Design review of the part shown in the three views and the two pictorial views. Dimensions are in mm from the part's minimum x, y and z. A direction names the side the tool comes from. Coordinates: 2 decimals unless noted, no trailing zeros. Loops run counter-clockwise (first coordinate to the right, second up) from the corner with the lowest first, then second, coordinate; pieces in that order, holes last. Notation, with made-up numbers: M 14.5,-31.75 L 56.5,-31.75 A19 ccw 56.5,-11.75 Z; hole C 17.5,41 d9. An arc over 180 degrees is marked long. Answer as a JSON object with one key per item and string values. Group by question number.
Item 1: Insertion check: pin 1 (2 mm diameter, centred on y = 3, z = 9.5, fed in from -X); pin 2 (2.5 mm diameter, centred on y = 5, z = 23, fed in from +X); pin 3 (3 mm diameter, centred on y = 4, z = 5, fed in from -X). Each pin has a flat end and moves straight along its axis. Give the tip position at first contact, or say it passes through.
Item 2: Add section C-C (z = 20). State the section outline as (x, y) points.
Item 3: Wall thickness on L1, parallel to Z at x = 20, y = 3; L2, parallel to Y at x = 20, z = 39.15; L3, parallel to X at y = 5.75, z = 14.5: over which ranges is each line inside the solid? List them lowest first. Write a range as from..to.
Item 4: Mouldability with a two-part tool opening along X and no side actions: class the marked faces 3 and 4 as +X half, -X half, draft (parallel to the pull), parting line (faces both ways), or undercut.
Item 5: Add section A-A (y = 4). State the section outline as (x, z) points (1 decimal).
Item 6: Add section D-D (z = 6.5). State the section outline as (x, y) points.
Item 7: Tool access review of the marked faces 1 and 2: name each direction out of +Z, -Z, +X, -X, +Y, -Y from which nothing blocks a thin tool from reaching the whole face with its end or side.
Item 8: Add section B-B (x = 20). State the section outline as (y, z) points, then the cut area to 3 significant figures.
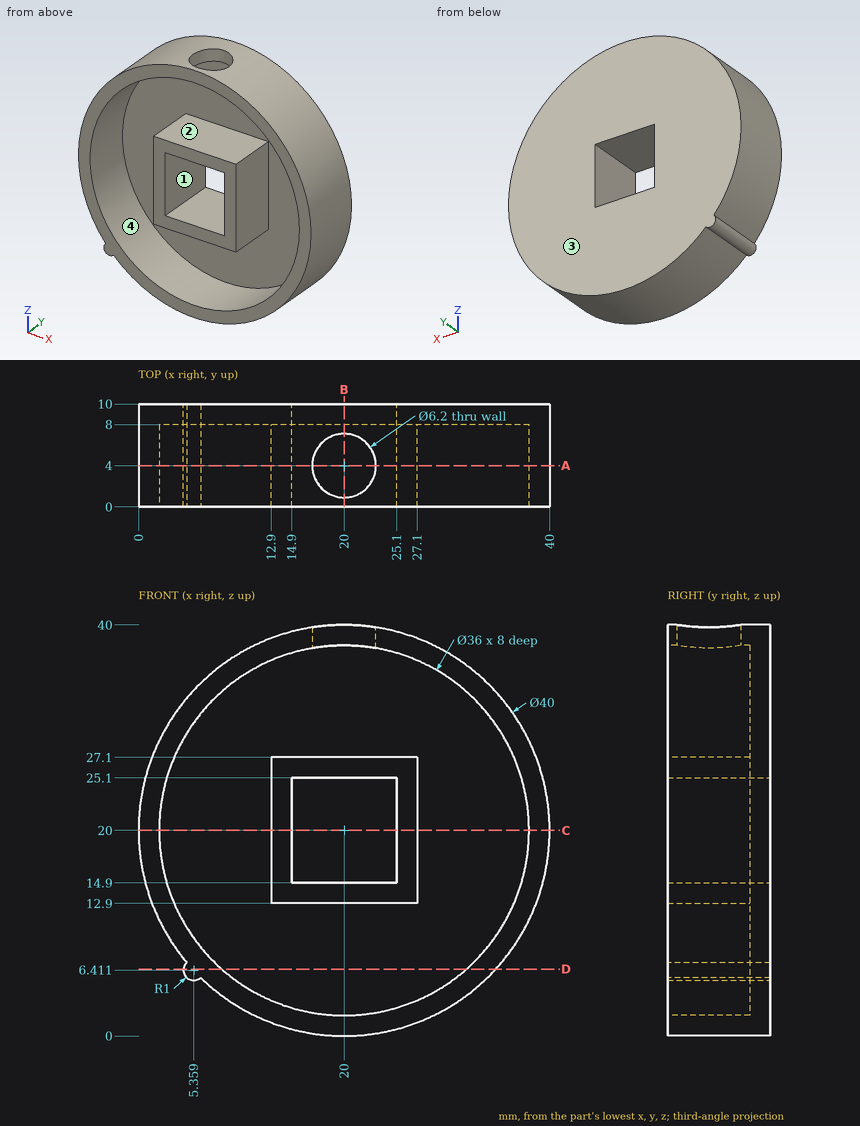
From the geometry:
{
 "1": {"pin 1": "stops at x = 2.4", "pin 2": "stops at x = 39.92", "pin 3": "stops at x = 4.36"},
 "2": {"outline": "M 0,0 L 2,0 L 2,8 L 12.9,8 L 12.9,0 L 14.9,0 L 14.9,10 L 0,10 Z; M 25.1,0 L 27.1,0 L 27.1,8 L 38,8 L 38,0 L 40,0 L 40,10 L 25.1,10 Z"},
 "3": {"L1": "z = 0..2, 12.9..14.9, 25.1..27.1", "L2": "y = 0..0.9, 7.1..10", "L3": "x = 0.77..2.86, 12.9..27.1, 37.14..39.23"},
 "4": {"face 3": "draft", "face 4": "undercut"},
 "5": {"outline": "M 4.7,7.1 A1 ccw 6,5.7 A20 ccw long 23.1,39.8 L 23.1,37.7 A18 cw long 16.9,37.7 L 16.9,39.8 A20 ccw Z; M 12.9,12.9 L 27.1,12.9 L 27.1,27.1 L 12.9,27.1 Z; hole M 14.9,14.9 L 25.1,14.9 L 25.1,25.1 L 14.9,25.1 Z"},
 "6": {"outline": "M 4.36,0 L 8.09,0 L 8.09,8 L 31.91,8 L 31.91,0 L 34.76,0 L 34.76,10 L 4.36,10 Z"},
 "7": {"face 1": "+Y, -Y", "face 2": "-Y"},
 "8": {"outline": "M 0,0 L 10,0 L 10,14.9 L 0,14.9 L 0,12.9 L 8,12.9 L 8,2 L 0,2 Z; M 0,25.1 L 10,25.1 L 10,40 L 7.1,40 L 7.1,38 L 8,38 L 8,27.1 L 0,27.1 Z; M 0,38 L 0.9,38 L 0.9,40 L 0,40 Z", "area": "111 mm²"}
}
